Model file for the job. Use its own axes, mm. Face numbers are marked on the shaded views. A direction names the side the tool comes from. Coordinates: 2 decimals unless noted, no trailing zeros. Loops run counter-clockwise (first coordinate to the right, second up) from the corner with the lowest first, then second, coordinate; pieces in that order, holes last. Notation, with made-up numbers: (-2.5, 51.25) -> (10.5, 51.25) arc R8 cw to (10.5, 55.25) -> close; hole circle Ø8 at (-25, 60.5). An arc over 180 degrees is marked (long way). Use one line per item in the form item = value.
```python
from build123d import *

# Parameters (mm, degrees)
F0_W      = 20
F0_H      = 40
F0_R      = 6.45
F0_R_2    = 2.825
F1_DEPTH  = 36.1
F2_W      = 20
F2_H      = 6.3
F3_DEPTH  = 7.3
F4_W      = 20
F4_H      = 6.3
F5_DEPTH  = 7.3
F6_DEPTH  = 41.2
F7_DEPTH  = 37.4
F9_W      = 20
F9_H      = 4.5
F10_DEPTH = 3.4
F8_R      = 1.3
F11_DEPTH = 8


with BuildPart() as f1:
    # F0 (on Top) → F1 (new body)
    with BuildSketch(Plane.XY):
        Rectangle(F0_W, F0_H)
        with Locations((0, 10.8)):
            Circle(F0_R, mode=Mode.SUBTRACT)
        with Locations((0, 10.8)):
            Circle(F0_R)
        with Locations((0, 10.8)):
            Circle(F0_R_2, mode=Mode.SUBTRACT)
        with Locations((0, 10.8)):
            Circle(F0_R_2)
    extrude(amount=F1_DEPTH)

    # F2 (on face) → F3 (join)
    with BuildSketch(Plane(origin=(0, 20, 0), x_dir=(-1, 0, 0), z_dir=(0, 1, 0))):
        with Locations((0, 26.85)):
            Rectangle(F2_W, F2_H)
    extrude(amount=F3_DEPTH)

    # F4 (on face) → F5 (join)
    with BuildSketch(Plane.XZ.offset(20)):
        with Locations((0, 26.858872)):
            Rectangle(F4_W, F4_H)
    extrude(amount=F5_DEPTH)

    # F0 (on Top) → F6 (join)
    with BuildSketch(Plane.XY):
        with Locations((0, 10.8)):
            Circle(F0_R_2)
    extrude(amount=F6_DEPTH)

    # F0 (on Top) → F7 (join)
    with BuildSketch(Plane.XY):
        with Locations((0, 10.8)):
            Circle(F0_R)
        with Locations((0, 10.8)):
            Circle(F0_R_2, mode=Mode.SUBTRACT)
    extrude(amount=F7_DEPTH)

    # F9 (on face) → F10 (cut)
    with BuildSketch(Plane.XY.offset(36.1)):
        with BuildLine():
            Line((-10, 20), (-10, 10.213363))
            ThreePointArc((-10, 10.213363), (-4e-06, 19.71317), (10, 10.213371))
            Line((10, 10.213371), (10, 20))
            Line((10, 20), (-10, 20))
        make_face()
        with Locations((0, -17.75)):
            Rectangle(F9_W, F9_H)
    extrude(amount=-F10_DEPTH, mode=Mode.SUBTRACT)

    # F8 (on face) → F11 (cut)
    with BuildSketch(Plane.XY.offset(30.008872)):
        with Locations((5.6, -24)):
            Circle(F8_R)
        with Locations((-5.6, -24)):
            Circle(F8_R)
        with Locations((5.6, 24)):
            Circle(F8_R)
        with Locations((-5.6, 24)):
            Circle(F8_R)
    extrude(amount=-F11_DEPTH, mode=Mode.SUBTRACT)


solid = f1.part
```
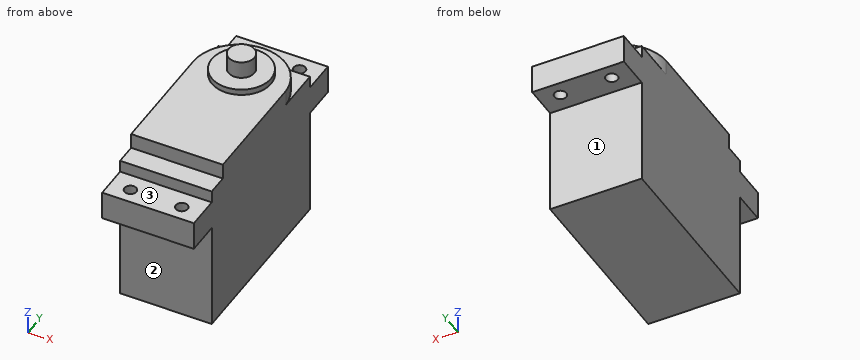
Q1. Band-saw the part on D-D, the plane y = 10.8. Write the cut outline in (x, z) (3 decimals), and give its area (3 significant figures).
Result:
outline = (-10, 0) -> (10, 0) -> (10, 32.7) -> (9.953, 32.7) -> (9.953, 36.1) -> (6.45, 36.1) -> (6.45, 37.4) -> (2.825, 37.4) -> (2.825, 41.2) -> (-2.825, 41.2) -> (-2.825, 37.4) -> (-6.45, 37.4) -> (-6.45, 36.1) -> (-9.953, 36.1) -> (-9.953, 32.7) -> (-10, 32.7) -> close
area = 760 mm2
Q2. Band-saw the part on A-A, the plane y = -24. Write the cut outline in (x, z), and give its area (3 significant figures).
Result:
outline = (-10, 23.71) -> (-6.9, 23.71) -> (-6.9, 30.01) -> (-10, 30.01) -> close; (-4.3, 23.71) -> (4.3, 23.71) -> (4.3, 30.01) -> (-4.3, 30.01) -> close; (6.9, 23.71) -> (10, 23.71) -> (10, 30.01) -> (6.9, 30.01) -> close
area = 93.2 mm2
Q3. Band-saw the part on B-B, the plane x = 5.6. Write the cut outline in (y, z), and give its area (3 significant figures).
Result:
outline = (-27.3, 23.71) -> (-25.3, 23.71) -> (-25.3, 30.01) -> (-27.3, 30.01) -> close; (-22.7, 23.71) -> (-20, 23.71) -> (-20, 0) -> (20, 0) -> (20, 23.7) -> (22.7, 23.7) -> (22.7, 30) -> (20, 30) -> (20, 32.7) -> (18, 32.7) -> (18, 36.1) -> (14, 36.1) -> (14, 37.4) -> (7.6, 37.4) -> (7.6, 36.1) -> (-15.5, 36.1) -> (-15.5, 32.7) -> (-20, 32.7) -> (-20, 30.01) -> (-22.7, 30.01) -> close; (25.3, 23.7) -> (27.3, 23.7) -> (27.3, 30) -> (25.3, 30) -> close
area = 1,490 mm2
Q4. Band-saw the part on C-C, the plane x = 0. Write the cut outline in (y, z) (3 decimals).
Result:
outline = (-27.3, 23.709) -> (-20, 23.709) -> (-20, 0) -> (20, 0) -> (20, 23.7) -> (27.3, 23.7) -> (27.3, 30) -> (20, 30) -> (20, 32.7) -> (19.713, 32.7) -> (19.713, 36.1) -> (17.25, 36.1) -> (17.25, 37.4) -> (13.625, 37.4) -> (13.625, 41.2) -> (7.975, 41.2) -> (7.975, 37.4) -> (4.35, 37.4) -> (4.35, 36.1) -> (-15.5, 36.1) -> (-15.5, 32.7) -> (-20, 32.7) -> (-20, 30.009) -> (-27.3, 30.009) -> close
Q5. Pin check, flat tips, straight feed: pin 1 Ø3.5 at (x, y) = (2.5, 23.5) entering from +Z; pin 2 Ø1 at (x, y) = (-2.5, 13.5) entering from +Z; pin 3 Ø1 at (x, z) = (4, 33.5) entering from -Y; pin 4 Ø2.5 at (x, y) = (-5.6, 24) entering from +Z. Stop position of each tip, or through.
Result:
pin_1 = 30
pin_2 = 37.4
pin_3 = -15.5
pin_4 = through
Q6. Wall check: line 1 along Y through (x, z) = (-5.6, 28.25); line 2 along X through (y, z) = (-23, 28); line 3 along Z through (x, y) = (-1.25, 2.5). Give the ranges that are in metal, low to high.
Result:
line_1 = -27.3 to -25.3, -22.7 to 22.7, 25.3 to 27.3
line_2 = -10 to -6.43, -4.77 to 4.77, 6.43 to 10
line_3 = 0 to 36.1
Q7. Which spindle directions (+Z, -Z, +X, -X, +Y, -Y) get a long thin tool onto all of the face, cutting with end or side? Do the marked faces 1, 2 and 3. Say none if no direction does.
Result:
face_1 = -Z, +X, -X, +Y
face_2 = -Z, +X, -X, -Y
face_3 = +Z, +X, -X, -Y
